Part print with two shaded views. Sizes in mm from the minimum x, y, z corner. A direction names the side the tool comes from. Coordinates: 2 decimals unless noted, no trailing zeros. Write each loop counter-clockwise with the first axis right and the second up, starting at its lowest first coordinate (ties: lowest second). Pieces come first, ordered by that corner, then holes.
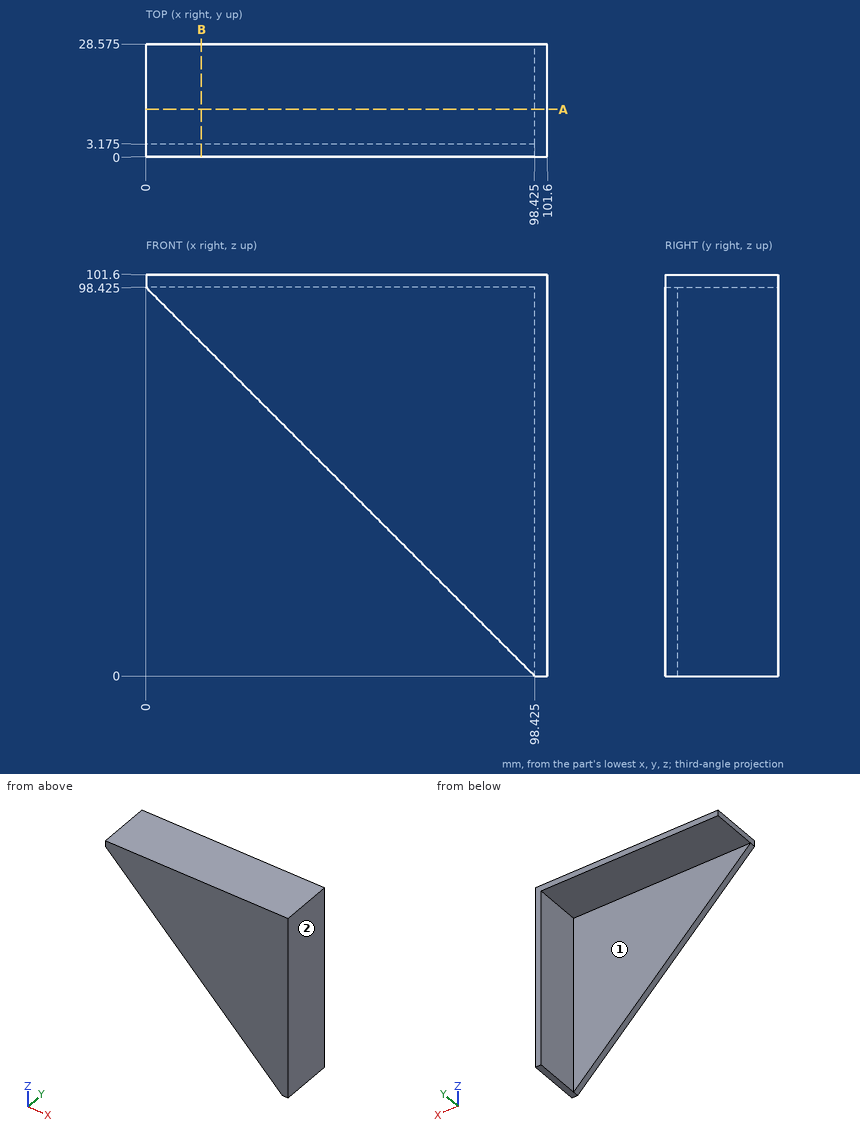
(1) 3-axis set-ups, long thin cutter, end or side, ignore diameter. For the marked faces 1 and 2: which of +Z, -Z, +X, -X, +Y, -Y reach the whole face in a straight line?
(2) Slice it at A-A, the plane y = 12. List the corners of the cut face in (x, z) (3 decimals), and give its area (3 significant figures).
(3) Probe L1, parallel to Z at x = 61, y = 8.5 (3 decimals); L2, parallel to Y at x = 24, z = 76 (3 decimals). List the from-to ranges inside material, lowest first.
(4) Slice it at B-B, the plane x = 14. List the corners of the cut face in (y, z) (3 decimals), and give its area (3 significant figures).
(5) Flat gauge pins, fed straight in: P1, Ø12, axis at x = 63, z = 51.5, coming from the +Y side (3 decimals); P2, Ø10, axis at x = 35, y = 20.5, coming from the -Z side (3 decimals); P3, Ø6, axis at y = 9.5, z = 53.5, coming from the -X side (3 decimals). Where does each tip first touch, or does it go through?
Results:
1. face 1: -Z, -X, +Y
1. face 2: +Z, -Z, +X, +Y, -Y
2. outline: (0, 98.425) - (98.425, 98.425) - (98.425, 0) - (101.6, 0) - (101.6, 101.6) - (0, 101.6) - close
2. area: 635 mm2
3. L1: z = 98.425 to 101.6
3. L2: y = 0 to 3.175
4. outline: (0, 84.425) - (3.175, 84.425) - (3.175, 98.425) - (28.575, 98.425) - (28.575, 101.6) - (0, 101.6) - close
4. area: 135 mm2
5. P1: stops at y = 3.175
5. P2: stops at z = 98.425
5. P3: stops at x = 98.425
